Geometry check sheet. Reference: drawing and pictorial views, mm from the part's lowest x, y, z. A direction names the side the tool comes from. Round coordinates to 2 decimals unless told otherwise and drop trailing zeros. Write each loop counter-clockwise with the first axis right and the second up, starting at its lowest first coordinate (ties: lowest second). Pieces come first, ordered by that corner, then holes. Notation, with made-up numbers: (26.5, 37.5) -> (41.5, 37.5) arc R33 cw to (41.5, 66.5) -> close; hole circle Ø6 at (55.25, 44). An arc over 180 degrees is marked (long way). Answer as a JSON object with one key per item and string values. Group by question number.
(1) Sectioned sample at D-D on z = 24.5. Record the cut outline in (x, y) (1 decimal), and give its area (3 significant figures).
(2) Draft check along X on the marked faces 6, 7, 8 and 9. Enter one of: released by +X, released by -X, zero draft, split by the parting line, or undercut.
(3) Set-up check for the marked faces 1, 2, 3, 4 and 5: record each of +Z, -Z, +X, -X, +Y, -Y from which the full face is reachable in a straight line by a thin tool's end or side.
(4) Sectioned sample at B-B on z = 20. Record the cut outline in (x, y) (1 decimal).
(5) Scan lines: L1, parallel to X at y = 11.75, z = 18; L2, parallel to X at y = 16.25, z = 11.5 (1 decimal); L3, parallel to Z at x = 13, y = 3. Record each from-to range of solid material in increasing order. Write a range as from..to.
(6) Sectioned sample at A-A on y = 6. Count the separate pieces of the cut face and the enclosed holes in it, and give its area (3 significant figures).
(7) Gauge pin test, flat ends, axial feed: pin 1 Ø5 at (x, y) = (15, 14.5) entering from +Z; pin 2 Ø1 at (x, z) = (21, 13.5) entering from +Y; pin 3 Ø10 at (x, y) = (34.5, 3) entering from +Z (3 decimals); pin 4 Ø1.5 at (x, y) = (53, 7) entering from +Z. Record the tip position at first contact, or that the pin passes through.
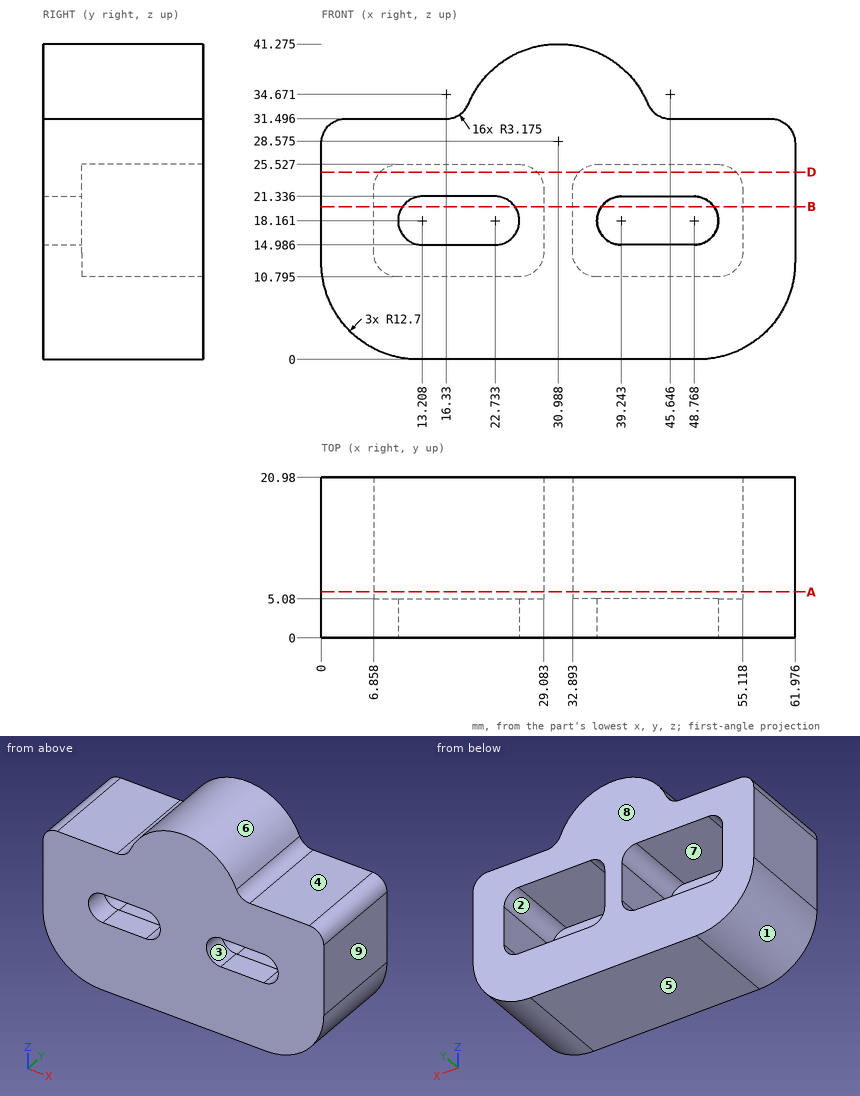
Computed values:
{
 "1": {"outline": "(0, 0) -> (62, 0) -> (62, 21) -> (54.3, 21) -> (54.3, 5.1) -> (33.7, 5.1) -> (33.7, 21) -> (28.2, 21) -> (28.2, 5.1) -> (7.7, 5.1) -> (7.7, 21) -> (0, 21) -> close", "area": "647 mm2"},
 "2": {"face 6": "split by the parting line", "face 7": "undercut", "face 8": "zero draft", "face 9": "released by +X"},
 "3": {"face 1": "-Z, -X, +Y, -Y", "face 2": "+Y", "face 3": "+Y, -Y", "face 4": "+Z, +X, +Y, -Y", "face 5": "-Z, +X, -X, +Y, -Y"},
 "4": {"outline": "(0, 0) -> (10.6, 0) -> (10.6, 5.1) -> (6.9, 5.1) -> (6.9, 21) -> (0, 21) -> close; (25.3, 0) -> (36.7, 0) -> (36.7, 5.1) -> (32.9, 5.1) -> (32.9, 21) -> (29.1, 21) -> (29.1, 5.1) -> (25.3, 5.1) -> close; (51.4, 0) -> (62, 0) -> (62, 21) -> (55.1, 21) -> (55.1, 5.1) -> (51.4, 5.1) -> close"},
 "5": {"L1": "0..6.86, 29.08..32.89, 55.12..61.98", "L2": "0.1..8, 27.9..34.1, 53.9..61.9", "L3": "0..14.99, 21.33..31.5"},
 "6": {"separate pieces": "1", "enclosed holes": "2", "area": "1,420 mm2"},
 "7": {"pin 1": "z = 31.72", "pin 2": "y = 5.08", "pin 3": "z = 41.275", "pin 4": "z = 31.5"}
}
